Could you check a few things on this drawing? It's one solid part, dimensions in mm from its lowest x, y, z. A direction names the side the tool comes from. Round coordinates to 2 decimals unless told otherwise and drop trailing zeros. Write each loop counter-clockwise with the first axis right and the second up, starting at its lowest first coordinate (ties: lowest second). Pieces come first, ordered by that corner, then holes. Notation, with made-up numbers: (57.25, -19) -> (95.25, -19) arc R25 ccw to (95.25, 1) -> close; hole circle Ø4 at (69.5, -23.75). An arc over 180 degrees is marked (long way). Return JSON: item names as keys, results as strings.
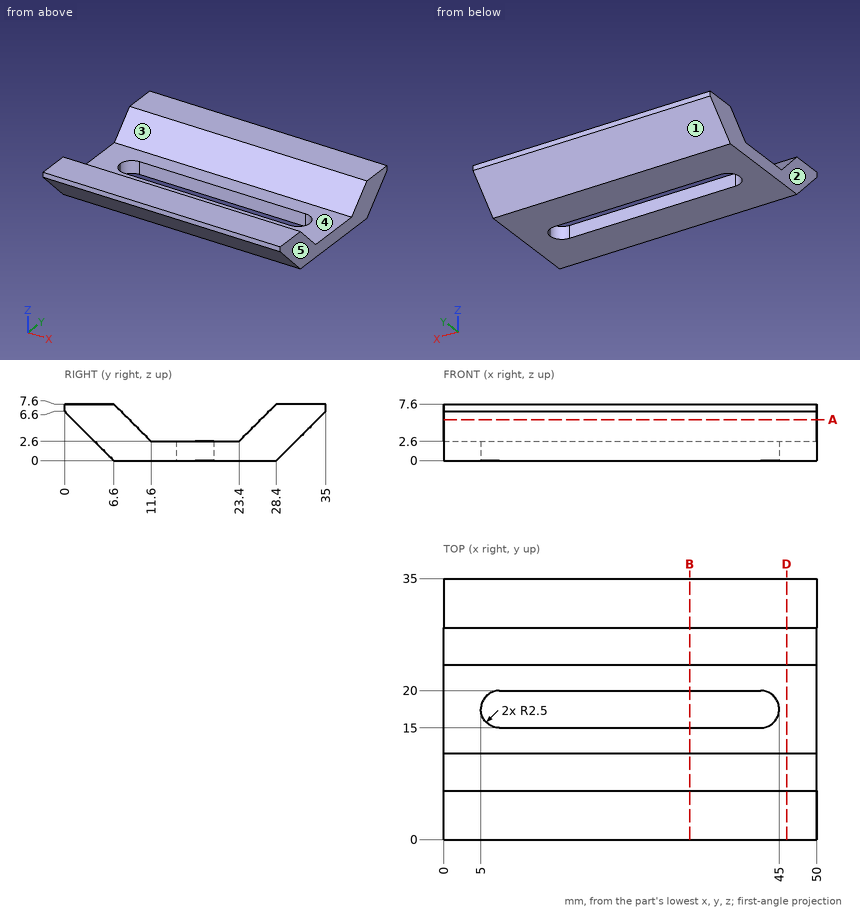
1) For the marked faces 4 and 5, which set-ups out of +Z, -Z, +X, -X, +Y, -Y let a thin tool reach every point of the face, with its end or its side?
Return value:
{"face 4": "+Z, +X, -X", "face 5": "+Z, -Z, +X, +Y, -Y"}
2) Thinking about a two-plate mould opening in Y: for the marked faces 1, 2 and 3, which applies, pulls with the +Y half, pulls with the -Y half, needs draft (parallel to the pull), parting line crosses it, or undercut?
Return value:
{"face 1": "pulls with the +Y half", "face 2": "needs draft", "face 3": "undercut"}
3) I want a section at D-D, the plane x = 46. Please give me the cut outline in (y, z).
Return value:
{"outline": "(0, 6.6) -> (6.6, 0) -> (28.4, 0) -> (35, 6.6) -> (35, 7.6) -> (28.4, 7.6) -> (23.4, 2.6) -> (11.6, 2.6) -> (6.6, 7.6) -> (0, 7.6) -> close"}
4) I want a section at B-B, the plane x = 33. Please give me the cut outline in (y, z), and give its area (3 significant figures).
Return value:
{"outline": "(0, 6.6) -> (6.6, 0) -> (15, 0) -> (15, 2.6) -> (11.6, 2.6) -> (6.6, 7.6) -> (0, 7.6) -> close; (20, 0) -> (28.4, 0) -> (35, 6.6) -> (35, 7.6) -> (28.4, 7.6) -> (23.4, 2.6) -> (20, 2.6) -> close", "area": "125 mm²"}
5) If I drill on probe 1 along Y at (x, z) = (9, 5.5); probe 2 along Y at (x, z) = (23, 6.75); probe 3 along Z at (x, y) = (38.5, 14), over which ranges is the centre line in solid material (lowest first)? Write a range as [from, to].
Return value:
{"probe 1": "[1.1, 8.7], [26.3, 33.9]", "probe 2": "[0, 7.45], [27.55, 35]", "probe 3": "[0, 2.6]"}
6) Will these pins go through, and if not, where does the flat tip stop? pin 1 Ø0.8 at (x, z) = (18.5, 1) entering from +Y; pin 2 Ø3 at (x, z) = (28.5, 3.5) entering from -Y; pin 3 Ø1.3 at (x, z) = (33.5, 1.5) entering from -Y; pin 4 Ø4 at (y, z) = (23, 6.5) entering from +X.
Return value:
{"pin 1": "y = 29.8", "pin 2": "y = 1.6", "pin 3": "y = 4.45", "pin 4": "through"}
7) I want a section at A-A, the plane z = 5.5. Please give me the cut outline in (x, y).
Return value:
{"outline": "(0, 1.1) -> (50, 1.1) -> (50, 8.7) -> (0, 8.7) -> close; (0, 26.3) -> (50, 26.3) -> (50, 33.9) -> (0, 33.9) -> close"}
